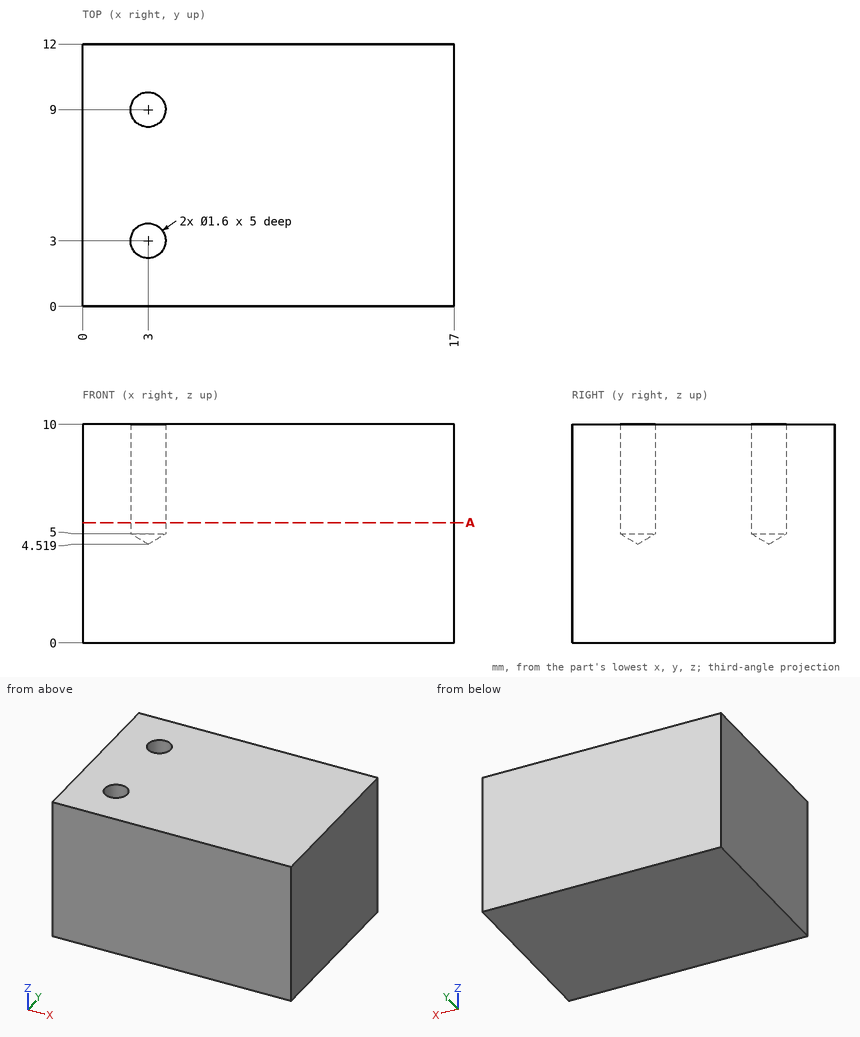
Here's the drawing with two shaded views (mm, measured from the low corner). I have some questions. Coordinates: 2 decimals unless noted, no trailing zeros. Loops run counter-clockwise (first coordinate to the right, second up) from the corner with the lowest first, then second, coordinate; pieces in that order, holes last. Notation, with made-up numbers: M 65,2 L 99,2 A18 cw 99,29 Z; hole C -37,56 d6. An arc over 180 degrees is marked long. Put each result on its own line as item: value. Start each with the question number.
(1) I need wall thicknesses on probe 1 along Y at (x, z) = (3, 7.25); probe 2 along X at (y, z) = (3, 8.55). Which ranges of each line are inside material? Lowest first, please.
(2) Imagine slicing it at A-A on z = 5.5. List the corners of the cut face in (x, y) for me, and give its area (3 significant figures).
(3) Will these pins go through, and if not, where does the flat tip stop? pin 1 Ø1.4 at (x, y) = (3, 3) entering from +Z; pin 2 Ø1 at (x, y) = (3, 9) entering from +Z.
Worked answers:
1. probe 1: y = 0 to 2.2, 3.8 to 8.2, 9.8 to 12
1. probe 2: x = 0 to 2.2, 3.8 to 17
2. outline: M 0,0 L 17,0 L 17,12 L 0,12 Z; hole C 3,3 d1.6; hole C 3,9 d1.6
2. area: 200 mm2
3. pin 1: stops at z = 4.94
3. pin 2: stops at z = 4.82
